Can you work these out from the model? Positions are in its coordinate system, mm. A direction names the side the tool comes from. Round coordinates to 2 decimals unless told otherwise and drop trailing zeros. Order: outer loops, then holes, each group sorted by start corner. A loop starts at its lowest first (then second) coordinate and runs counter-clockwise, first axis right, second up. Notation, with made-up numbers: (-4, 2.25) -> (25, 2.25) arc R21 cw to (25, 11.25) -> close; hole circle Ø8 at (35.25, 51). An arc over 180 degrees is marked (long way). One line per item, written item: value.
```python
from build123d import *

# Parameters (mm, degrees)
F0_R            = 38.1
F1_DEPTH        = 25.4
F3_DEPTH        = 25.4
F3_COPIES_COUNT = 30


# Not quite as in the source:
# - a pattern or mirror of a feature is missing from the dataset's text; its kind, count and spacing are read off the source's solid


with BuildPart() as f1:
    # F0 (on Front) → F1 (new body)
    with BuildSketch(Plane.XZ):
        Circle(F0_R)
    extrude(amount=F1_DEPTH)

    # F2 (on face) → F3 (join)
    with BuildSketch(Plane.XZ.offset(25.4)):
        with BuildLine():
            Line((1.8707504496, 42.7830666304), (-2.323463975, 38.0290877508))
            ThreePointArc((-2.323463975, 38.0290877508), (1.6643863058, 38.0636285478), (5.6340012219, 37.6811362651))
            Line((5.6340012219, 37.6811362651), (1.8707504496, 42.7830666304))
        make_face()
    f3 = extrude(amount=-F3_DEPTH)

    # F3_copies: F3 ×30 about axis
    f3_copies_axis = Axis((0, 0, 0), (0, 1, 0))
    for i in range(1, F3_COPIES_COUNT):
        add(f3.rotate(f3_copies_axis, i * 360 / F3_COPIES_COUNT))


solid = f1.part
```
Q1. I want a section at B-B on z = -26. List the corners of the cut face in (x, y) for me.
Answers below:
outline: (-32.79, -25.4) -> (30.08, -25.4) -> (30.08, 0) -> (-32.79, 0) -> close
Q2. I want a section at A-A on x = 8.5. List the corners of the cut face in (y, z) for me.
Answers below:
outline: (-25.4, -39.69) -> (0, -39.69) -> (0, 39.81) -> (-25.4, 39.81) -> close
Q3. On a 3-axis mill with a long thin cutter (end or side, diameter ignored), from which of +Z, -Z, +X, -X, +Y, -Y can I reach the whole of each face in a straight line? I mean faces 4 (the face through (-32.4, -12.88, -24.09)), 5 (the face through (-8.22, -12.88, -39.6)), 6 (the face through (-16.63, -12.88, 36.86)), 7 (the face through (40.37, -12.88, 0.44)). Say none if no direction works.
Answers below:
face 4: -X, +Y, -Y
face 5: -Z, +Y, -Y
face 6: +Z, +Y, -Y
face 7: +X, +Y, -Y
Q4. Will these pins go through, and if not, where does the flat tip stop? pin 1 Ø6 at (x, y) = (28.5, -4) entering from +Z; pin 2 Ø5 at (y, z) = (-3.5, 33.5) entering from -X; pin 3 Ø8 at (y, z) = (-22, 34) entering from +X.
Answers below:
pin 1: z = 33.51
pin 2: x = -24.08
pin 3: x = 26.69
Q5. Please list where these lines run through material, in increasing order: line 1 along Z through (x, y) = (-10.5, -21.5); line 2 along Z through (x, y) = (-18.5, -8.25); line 3 along X through (y, z) = (-13.5, -8).
Answers below:
line 1: -41.29 to 36.9
line 2: -38.04 to 34.08
line 3: -38.8 to 39.51
Q6. We'd pull the mould along X, two halves only. Please class faces 1 (the face through (23.61, -12.88, 32.83)), 2 (the face through (-34.92, -12.88, -20.39)), 3 (the face through (35.12, -12.88, -20.05)): released by +X, released by -X, zero draft, split by the parting line, or undercut.
Answers below:
face 1: undercut
face 2: released by -X
face 3: released by +X
